Answer from the drawing. Dimensions are ordinates in mm from the lowest x, y and z of the part. A direction names the side the tool comes from. Coordinates: 2 decimals unless noted, no trailing zeros. Write each loop counter-clockwise with the first axis right and the second up, starting at its lowest first coordinate (ties: lowest second). Pieces come first, ordered by that corner, then holes. Notation, with made-up numbers: (83, 17.5) -> (100, 17.5) arc R18 ccw to (100, 52.5) -> close; hole circle Ø6 at (-15, 43). An arc over 180 degrees is marked (long way). Return JSON: item names as keys, results as strings.
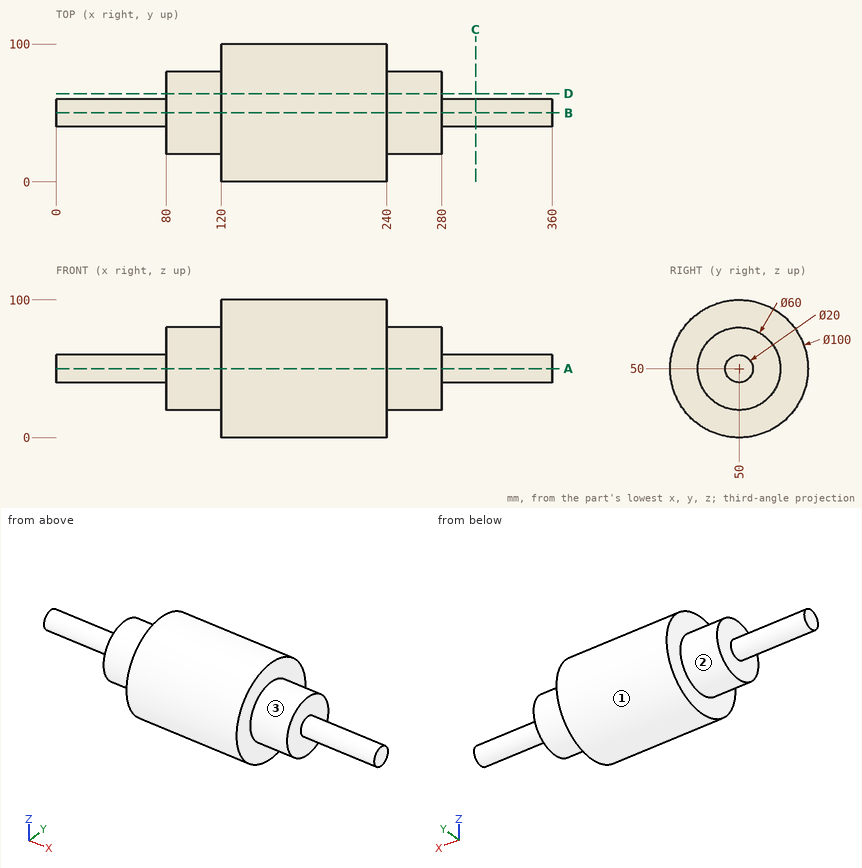
1. A tool of negligible diameter and unlimited length cuts with its end or side. For the marked faces 1, 2 and 3, from which of +Z, -Z, +X, -X, +Y, -Y can it reach the whole face along a straight path? Write none if from no direction.
Taken from the geometry:
{"face 1": "+X, -X", "face 2": "-X", "face 3": "+X"}
2. The part is cut by section D-D (y = 64). Determine the outline of the cut face in (x, z), then the cut area to 3 significant figures.
Taken from the geometry:
{"outline": "(80, 23.47) -> (120, 23.47) -> (120, 2) -> (240, 2) -> (240, 23.47) -> (280, 23.47) -> (280, 76.53) -> (240, 76.53) -> (240, 98) -> (120, 98) -> (120, 76.53) -> (80, 76.53) -> close", "area": "15,800 mm2"}
3. Consider L1, parallel to X at y = 55, z = 7.5; L2, parallel to Y at x = 169.5, z = 81; L3, parallel to Y at x = 213, z = 75. Determine where each line is inside the solid, lowest interval first.
Taken from the geometry:
{"L1": "x = 120 to 240", "L2": "y = 10.77 to 89.23", "L3": "y = 6.7 to 93.3"}
4. Flat-ended cylindrical pins translate along their axes: pin 1 Ø5 at (y, z) = (26, 71.5) entering from -X; pin 2 Ø10 at (x, z) = (87.5, 24.5) entering from +Y; pin 3 Ø5 at (x, z) = (290.5, 55) entering from +Y; pin 4 Ø8 at (x, y) = (318.5, 35.5) entering from -Z. Find the tip coordinate at first contact, or state that the pin passes through.
Taken from the geometry:
{"pin 1": "stops at x = 80", "pin 2": "stops at y = 71.9", "pin 3": "stops at y = 59.68", "pin 4": "passes through"}
5. The part is cut by section C-C (x = 304.5). Determine the outline of the cut face in (y, z), then the cut area to 3 significant figures.
Taken from the geometry:
{"outline": "circle Ø20 at (50, 50)", "area": "314 mm2"}
6. The part is cut by section A-A (z = 50). Determine the outline of the cut face in (x, y).
Taken from the geometry:
{"outline": "(0, 40) -> (80, 40) -> (80, 20) -> (120, 20) -> (120, 0) -> (240, 0) -> (240, 20) -> (280, 20) -> (280, 40) -> (360, 40) -> (360, 60) -> (280, 60) -> (280, 80) -> (240, 80) -> (240, 100) -> (120, 100) -> (120, 80) -> (80, 80) -> (80, 60) -> (0, 60) -> close"}
